Could you check a few things on this model? Use its own coordinates, in mm. Face numbers are marked on the shaded views. A direction names the side the tool comes from. Round coordinates to 2 decimals unless told otherwise and drop trailing zeros. Loops run counter-clockwise (first coordinate to the right, second up) from the corner with the lowest first, then second, coordinate; pieces in that order, holes last. Notation, with made-up numbers: M 70.5,63 L 108.5,63 A18 cw 108.5,67 Z; hole C 29,5.5 d2. An arc over 180 degrees is marked long. Answer in a Markdown table with one row per item.
```python
from build123d import *

# Parameters (mm, degrees)
F0_W     = 50.8
F0_H     = 50.8
F1_DEPTH = 74.224433
F2_R     = 12.7
F3_DEPTH = 25.4
F4_W     = 101.6
F4_H     = 76.2
F5_DEPTH = 127


with BuildPart() as f1:
    # F0 (on Top) → F1 (new body)
    with BuildSketch(Plane.XY):
        Rectangle(F0_W, F0_H)
    extrude(amount=F1_DEPTH)

    # F2 (on face) → F3 (join)
    with BuildSketch(Plane(origin=(-25.4, 0, 0), x_dir=(0, -1, 0), z_dir=(-1, 0, 0))):
        with Locations((0, 37.112216)):
            Circle(F2_R)
    extrude(amount=F3_DEPTH)

    # F4 (on face) → F5 (join)
    with BuildSketch(Plane.XZ.offset(25.4)):
        with Locations((0, 37.112216)):
            Rectangle(F4_W, F4_H)
    extrude(amount=F5_DEPTH)


solid = f1.part
```
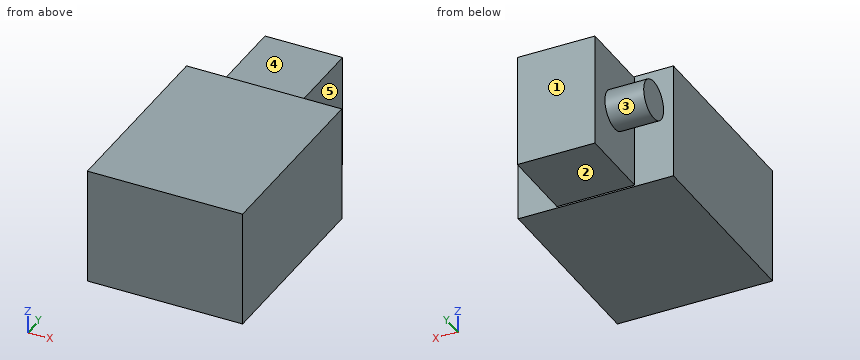
1) I want a section at D-D, the plane x = 36.5. Please give me the cut outline in (y, z).
Computed:
| item | result |
|---|---|
| outline | M -152.4,-0.99 L -25.4,-0.99 L -25.4,75.21 L -152.4,75.21 Z |
2) Which directions (+Z, -Z, +X, -X, +Y, -Y) give clear straight access to the entire face, cutting with the end or side of a thin tool? Please do the marked faces 1, 2, 3, 4 and 5.
Computed:
| item | result |
|---|---|
| face 1 | +Z, -Z, +X, -X, +Y |
| face 2 | -Z, +X, -X, +Y |
| face 3 | -X |
| face 4 | +Z, +X, -X, +Y |
| face 5 | +Z, -Z, +X, +Y |
3) I want a section at B-B, the plane x = -41. Please give me the cut outline in (y, z).
Computed:
| item | result |
|---|---|
| outline | M -152.4,-0.99 L -25.4,-0.99 L -25.4,75.21 L -152.4,75.21 Z; C 0,37.11 d25.4 |
4) I want a section at C-C, the plane y = 0. Please give me the cut outline in (x, z), plus the area to 3 significant figures.
Computed:
| item | result |
|---|---|
| outline | M -50.8,24.41 L -25.4,24.41 L -25.4,0 L 25.4,0 L 25.4,74.22 L -25.4,74.22 L -25.4,49.81 L -50.8,49.81 Z |
| area | 4,420 mm² |
5) I want a section at A-A, the plane z = 5.5. Please give me the cut outline in (x, y), plus the area to 3 significant figures.
Computed:
| item | result |
|---|---|
| outline | M -50.8,-152.4 L 50.8,-152.4 L 50.8,-25.4 L 25.4,-25.4 L 25.4,25.4 L -25.4,25.4 L -25.4,-25.4 L -50.8,-25.4 Z |
| area | 15,500 mm² |
6) I need wall thicknesses on line 1 (X direction, y = 15, z = 10.5); line 2 (Y direction, x = 40.5, z = 67.5); line 3 (Y direction, x = -30, z = 43.5). Which ranges of each line are inside material? Lowest first, please.
Computed:
| item | result |
|---|---|
| line 1 | x = -25.4 to 25.4 |
| line 2 | y = -152.4 to -25.4 |
| line 3 | y = -152.4 to -25.4, -10.98 to 10.98 |
7) Will these pins go through, and if not, where does the flat tip stop? P1, Ø10, axis at x = 36, z = 41, coming from the +Y side; P2, Ø15, axis at y = 9.5, z = 52, coming from the +X side.
Computed:
| item | result |
|---|---|
| P1 | stops at y = -25.4 |
| P2 | stops at x = 25.4 |
